from build123d import *

# Parameters (mm, degrees)
F0_R     = 2.55
F0_W     = 26
F0_H     = 15
F0_R_2   = 4
F1_DEPTH = 4


with BuildPart() as f1:
    # F0 (on Front) → F1 (new body)
    with BuildSketch(Plane.XZ):
        with BuildLine():
            Line((-17.5, 95.5), (-17.5, 5))
            ThreePointArc((-17.5, 5), (-16.035534, 1.464466), (-12.5, 0))
            Line((-12.5, 0), (25.5, 0))
            ThreePointArc((25.5, 0), (29.035534, 1.464466), (30.5, 5))
            Line((30.5, 5), (30.5, 95.5))
            ThreePointArc((30.5, 95.5), (29.035534, 99.035534), (25.5, 100.5))
            Line((25.5, 100.5), (-12.5, 100.5))
            ThreePointArc((-12.5, 100.5), (-16.035534, 99.035534), (-17.5, 95.5))
        make_face()
        with Locations((12.5, 10)):
            Circle(F0_R, mode=Mode.SUBTRACT)
        with Locations((12.5, 25.05)):
            Rectangle(F0_W, F0_H, mode=Mode.SUBTRACT)
        with Locations((-2.5, 68)):
            Circle(F0_R_2, mode=Mode.SUBTRACT)
        with Locations((12.5, 88)):
            Circle(F0_R_2, mode=Mode.SUBTRACT)
    extrude(amount=F1_DEPTH)


solid = f1.part
Could you check a few things on this model? Use its own coordinates, in mm. A direction names the side the tool comes from. Round coordinates to 2 decimals unless told otherwise and drop trailing zeros. Loops run counter-clockwise (first coordinate to the right, second up) from the corner with the lowest first, then second, coordinate; pieces in that order, holes last. Notation, with made-up numbers: (23, 27.25) -> (53, 27.25) arc R12 cw to (53, 48.25) -> close; hole circle Ø10 at (77, 23.5). An arc over 180 degrees is marked (long way). Use CSV: the item, a comma, the result in double quotes.
(1) Will this pin go through, and if not, where does the flat tip stop? pin 1 Ø6.5 at (x, z) = (-2.5, 68) entering from +Y.
Return value:
pin 1,"passes through"
(2) If we mould it in two halves opening along X, with no side actions, what happens to faces 1 (the flat face through (12, -2, 17.55)), 2 (the flat face through (6, -2, 0)), 3 (the cylindrical face through (29.07, -1.97, 99))? For each: +X half, -X half, draft (parallel to the pull), parting line (faces both ways), or undercut.
Return value:
face 1,"undercut"
face 2,"draft"
face 3,"+X half"
(3) Suppose I cut it at D-D on y = -0.6. Write out the boundary of the cut face in (x, z).
Return value:
outline,"(-17.5, 5) arc R5 ccw to (-12.5, 0) -> (25.5, 0) arc R5 ccw to (30.5, 5) -> (30.5, 95.5) arc R5 ccw to (25.5, 100.5) -> (-12.5, 100.5) arc R5 ccw to (-17.5, 95.5) -> close; hole circle Ø8 at (-2.5, 68); hole (-0.5, 17.55) -> (25.5, 17.55) -> (25.5, 32.55) -> (-0.5, 32.55) -> close; hole circle Ø8 at (12.5, 88); hole circle Ø5.1 at (12.5, 10)"
(4) Suppose I cut it at A-A on x = -2.5. Write out the boundary of the cut face in (y, z), plus the area to 3 significant figures.
Return value:
outline,"(-4, 0) -> (0, 0) -> (0, 64) -> (-4, 64) -> close; (-4, 72) -> (0, 72) -> (0, 100.5) -> (-4, 100.5) -> close"
area,"370 mm²"
(5) If I drill on probe 1 along Z at (x, y) = (12.5, -1.05); probe 2 along Z at (x, y) = (4, -2.55); probe 3 along Z at (x, y) = (-2.5, -2), over which ranges is the centre line in solid material (lowest first)? Write a range as [from, to].
Return value:
probe 1,"z = [0, 7.45], [12.55, 17.55], [32.55, 84], [92, 100.5]"
probe 2,"z = [0, 17.55], [32.55, 100.5]"
probe 3,"z = [0, 64], [72, 100.5]"
(6) For faces 4 (the flat face through (6, 0, 51)), 5 (the flat face through (25.5, -2, 25)), which set-ups out of +Z, -Z, +X, -X, +Y, -Y let a thin tool reach every point of the face, with its end or its side?
Return value:
face 4,"+Z, -Z, +X, -X, +Y"
face 5,"+Y, -Y"
(7) Suppose I cut it at C-C on x = 12.5. Write out the boundary of the cut face in (y, z).
Return value:
outline,"(-4, 0) -> (0, 0) -> (0, 7.45) -> (-4, 7.45) -> close; (-4, 12.55) -> (0, 12.55) -> (0, 17.55) -> (-4, 17.55) -> close; (-4, 32.55) -> (0, 32.55) -> (0, 84) -> (-4, 84) -> close; (-4, 92) -> (0, 92) -> (0, 100.5) -> (-4, 100.5) -> close"
(8) Suppose I cut it at B-B on z = 21.5. Write out the boundary of the cut face in (x, y), plus the area to 3 significant figures.
Return value:
outline,"(-17.5, -4) -> (-0.5, -4) -> (-0.5, 0) -> (-17.5, 0) -> close; (25.5, -4) -> (30.5, -4) -> (30.5, 0) -> (25.5, 0) -> close"
area,"88.0 mm²"
